```python
from build123d import *

# Parameters (mm, degrees)
F0_R      = 11.1
F1_DEPTH  = 30
F2_R      = 7.5
F3_DEPTH  = 20
F4_R      = 6
F5_DEPTH  = 17
F6_R      = 4.5
F7_DEPTH  = 2
F8_R      = 6
F9_DEPTH  = 23.5
F10_R     = 4.75
F11_DEPTH = 10


with BuildPart() as f1:
    # F0 (on Right) → F1 (new body)
    with BuildSketch(Plane.YZ):
        Circle(F0_R)
    extrude(amount=F1_DEPTH)

    # F2 (on face) → F3 (join)
    with BuildSketch(Plane.YZ.offset(30)):
        Circle(F2_R)
    extrude(amount=F3_DEPTH)

    # F4 (on face) → F5 (join)
    with BuildSketch(Plane.YZ.offset(50)):
        Circle(F4_R)
    extrude(amount=F5_DEPTH)

    # F6 (on face) → F7 (join)
    with BuildSketch(Plane.YZ.offset(67)):
        Circle(F6_R)
    extrude(amount=F7_DEPTH)

    # F8 (on face) → F9 (join)
    with BuildSketch(Plane.YZ.offset(69)):
        Circle(F8_R)
    extrude(amount=F9_DEPTH)

    # F10 (on face) → F11 (join)
    with BuildSketch(Plane.YZ.offset(92.5)):
        Circle(F10_R)
    extrude(amount=F11_DEPTH)


solid = f1.part
```
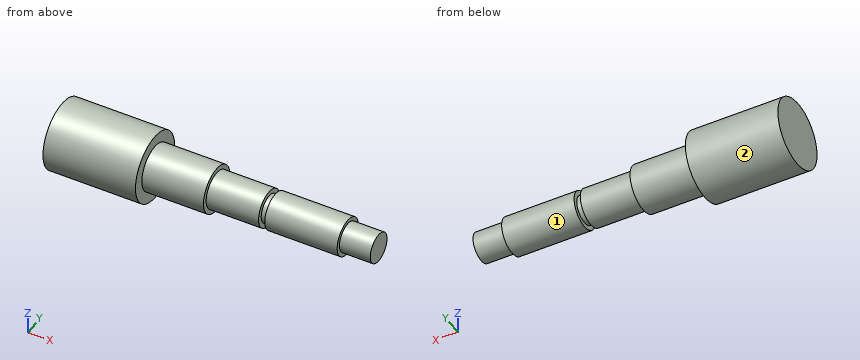
Can you work these out from the model? Positions are in its coordinate system, mm. Face numbers are marked on the shaded views. A direction names the side the tool comes from. Round coordinates to 2 decimals unless told otherwise and drop trailing zeros. Order: outer loops, then holes, each group sorted by start corner. A loop starts at its lowest first (then second) coordinate and runs counter-clockwise, first axis right, second up.
(1) I'm going to push flat-ended pins straight in: pin 1 (1.5 mm diameter, centred on y = 6, z = -2.5, fed in from +X); pin 2 (1 mm diameter, centred on x = 58, y = 1.5, fed in from -Z); pin 3 (10 mm diameter, centred on x = 13, y = -7, fed in from +Z); pin 4 (1 mm diameter, centred on y = -9, z = 8, fed in from +X). Where does each tip first touch, or does it pass through?
Results are:
pin 1: stops at x = 92.5
pin 2: stops at z = -5.92
pin 3: stops at z = 10.92
pin 4: passes through
(2) If we section it at A-A (y = 0): Please give me the cut outline in (x, z).
Results are:
outline: (0, -11.1) - (30, -11.1) - (30, -7.5) - (50, -7.5) - (50, -6) - (67, -6) - (67, -4.5) - (69, -4.5) - (69, -6) - (92.5, -6) - (92.5, -4.75) - (102.5, -4.75) - (102.5, 4.75) - (92.5, 4.75) - (92.5, 6) - (69, 6) - (69, 4.5) - (67, 4.5) - (67, 6) - (50, 6) - (50, 7.5) - (30, 7.5) - (30, 11.1) - (0, 11.1) - close
(3) On a 3-axis mill with a long thin cutter (end or side, diameter ignored), from which of +Z, -Z, +X, -X, +Y, -Y can I reach the whole of each face in a straight line? I mean the marked faces 1 and 2. Say none if no direction works.
Results are:
face 1: +X
face 2: +X, -X
(4) If I drill on L1, parallel to X at y = -4.75, z = -5.5; L2, parallel to X at y = -7.75, z = 6.5; L3, parallel to Y at x = 31, z = 6.75, over which ranges is the centre line in solid material (lowest first)?
Results are:
L1: x = 0 to 50
L2: x = 0 to 30
L3: y = -3.27 to 3.27
(5) If we section it at B-B (z = -2.75): Please give me the cut outline in (x, y), plus the area to 3 significant figures.
Results are:
outline: (0, -10.75) - (30, -10.75) - (30, -6.98) - (50, -6.98) - (50, -5.33) - (67, -5.33) - (67, -3.56) - (69, -3.56) - (69, -5.33) - (92.5, -5.33) - (92.5, -3.87) - (102.5, -3.87) - (102.5, 3.87) - (92.5, 3.87) - (92.5, 5.33) - (69, 5.33) - (69, 3.56) - (67, 3.56) - (67, 5.33) - (50, 5.33) - (50, 6.98) - (30, 6.98) - (30, 10.75) - (0, 10.75) - close
area: 1,450 mm2
(6) If we section it at D-D (x = 26): Please give me the cut outline in (y, z).
Results are:
outline: circle Ø22.2 at (0, 0)
(7) If we section it at C-C (x = 52): Please give me the cut outline in (y, z), plus the area to 3 significant figures.
Results are:
outline: circle Ø12 at (0, 0)
area: 113 mm2
